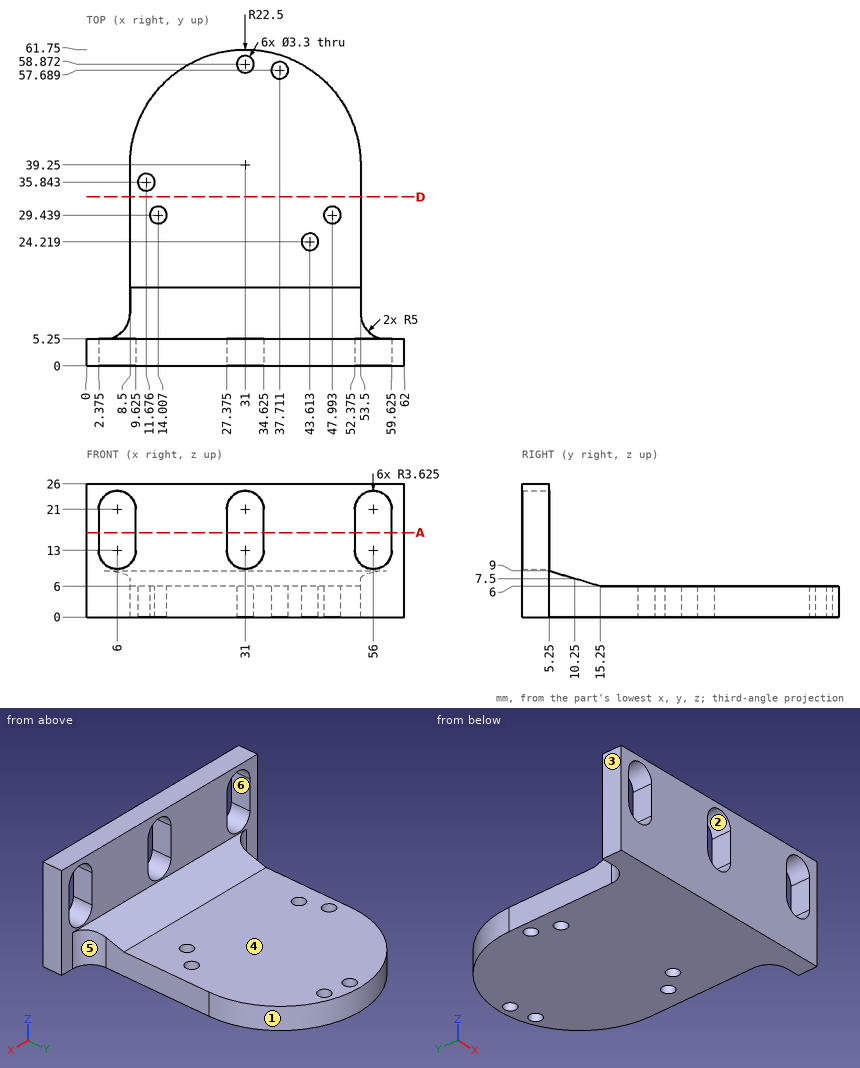
Geometry: see drawing. Coordinates: mm, zero at the bounding-box minimum. A direction names the side the tool comes from. Give positions to 0.01 mm unless a question says otherwise; leave off trailing zeros. Loops run counter-clockwise (first coordinate to the right, second up) from the corner with the lowest first, then second, coordinate; pieces in that order, holes last. Notation, with made-up numbers: (-8.5, 13) - (10.5, 13) arc R14 cw to (10.5, 22) - close; hole circle Ø11 at (-6.75, 41.5). An arc over 180 degrees is marked (long way). Use CSV: the item, a comma, the result in double quotes. Start each with the question number.
Item 1: Contact query for flat-ended pins moving along their axis: P1, Ø12, axis at y = 50, z = 9, coming from the +X side; P2, Ø10, axis at x = 44, z = 14, coming from the -Y side; P3, Ø2, axis at x = 37, y = 50.5, coming from the +Z side; P4, Ø2.5, axis at x = 37.71, y = 57.69, coming from the +Z side. Output: stop coordinate, or through.
Item 2: Section D-D on y = 33. Return loops of the section in (x, z), then the cut area to 3 significant figures.
Item 3: Line query: line 1 (Z direction, x = 24, y = 51); line 2 (Y direction, x = 34, z = 24.5); line 3 (Y direction, x = 13.5, z = 1.5). Output: solid intervals per line, ascending.
Item 4: Section A-A on z = 16.5. State how many separate pieces and enclosed holes the cut face has, then the cut area to 3 significant figures.
Item 5: Mould query, pull axis X, two halves, no side actions, for the marked faces 1, 2 and 3. Classes: pulls with the +X half, pulls with the -X half, needs draft (parallel to the pull), parting line crosses it, or undercut.
Item 6: Reachability of the marked faces 4, 5 and 6 from +Z, -Z, +X, -X, +Y, -Y: full face, straight path, thin tool, end or side. Return the list, or none.
Ans:
1,P1,"stops at x = 52.8"
1,P2,"stops at y = 0"
1,P3,"stops at z = 6"
1,P4,"passes through"
2,outline,"(8.5, 0) - (53.5, 0) - (53.5, 6) - (8.5, 6) - close"
2,area,"270 mm2"
3,line 1,"z = 0 to 6"
3,line 2,"y = 0 to 5.25"
3,line 3,"y = 0 to 27.87, 31.01 to 53.39"
4,separate pieces,"4"
4,enclosed holes,"0"
4,area,"211 mm2"
5,face 1,"parting line crosses it"
5,face 2,"undercut"
5,face 3,"pulls with the -X half"
6,face 4,"+Z, +X, -X, +Y"
6,face 5,"+Z, -Z, +X, +Y"
6,face 6,"+Y, -Y"
